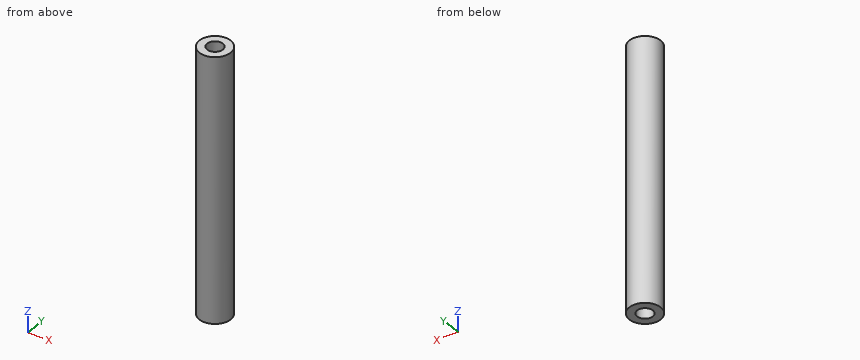
Autodesk Inventor part; units mm, degrees
ref_plane "作業平面1" through (0, 0, 44) normal (0, 0, 1) x (1, 0, 0)
ref_plane "YZ Plane" through (0, 0, 0) normal (1, 0, 0) x (0, 1, 0)
ref_plane "XZ Plane" through (0, 0, 0) normal (0, 1, 0) x (-1, 0, 0)
sketch "スケッチ1" plane through (0, 0, 0) normal (0, 0, 1) x (1, 0, 0)
  circle A0 centre (0, 0) radius 1.5
  circle A1 centre (0, 0) radius 3
  dimension "d0" = 3
  dimension "d1" = 6
extrude "押し出し1" add sketch "スケッチ1" along normal blind 50
ref_plane "作業平面1" through (0, 0, 44) normal (0, 0, 1) x (1, 0, 0)
sketch "スケッチ3" plane through (0, 0, 44) normal (0, 0, 1) x (1, 0, 0)
  circle A0 centre (0, 0) radius 1.5
extrude "押し出し3" add sketch "スケッチ3" against normal blind 38
properties part number "スペーサーm3,50" material "アルミニウム 7075"
Here's how the part is built. I have some questions about the finished solid (model axes, mm). Give positions to 0.01 mm unless a question says otherwise; leave off trailing zeros. Order: outer loops, then holes, each group sorted by start corner. A loop starts at its lowest first (then second) coordinate and runs counter-clockwise, first axis right, second up. Notation, with made-up numbers: (43.25, 70) -> (93.25, 70) arc R4 cw to (93.25, 75) -> close; hole circle Ø6 at (11.25, -18). An arc over 180 degrees is marked (long way). One line per item, written item: value. Start each with the question number.
1. I need wall thicknesses on probe 1 along Y at (x, z) = (0, 46.6); probe 2 along X at (y, z) = (0.25, 10.5); probe 3 along Z at (x, y) = (1.05, 0.1). Which ranges of each line are inside material? Lowest first, please. Write a range as from..to.
2. Imagine slicing it at C-C, the plane z = 41. List the corners of the cut face in (x, y) for me, plus the area to 3 significant figures.
3. Imagine slicing it at A-A, the plane x = 0. List the corners of the cut face in (y, z) for me, plus the area to 3 significant figures.
4. Will these pins go through, and if not, where does the flat tip stop? pin 1 Ø0.9 at (x, y) = (0, 0.5) entering from +Z; pin 2 Ø1 at (y, z) = (-2, 20) entering from +X; pin 3 Ø2 at (y, z) = (-1.5, 34.5) entering from -X.
5. Imagine slicing it at D-D, the plane x = -2.45. List the corners of the cut face in (y, z) for me, plus the area to 3 significant figures.
Values follow:
1. probe 1: y = -3..-1.5, 1.5..3
1. probe 2: x = -2.99..2.99
1. probe 3: z = 6..44
2. outline: circle Ø6 at (0, 0)
2. area: 28.3 mm2
3. outline: (-3, 0) -> (-1.5, 0) -> (-1.5, 6) -> (1.5, 6) -> (1.5, 0) -> (3, 0) -> (3, 50) -> (1.5, 50) -> (1.5, 44) -> (-1.5, 44) -> (-1.5, 50) -> (-3, 50) -> close
3. area: 264 mm2
4. pin 1: stops at z = 44
4. pin 2: stops at x = 2.6
4. pin 3: stops at x = -2.96
5. outline: (-1.73, 0) -> (1.73, 0) -> (1.73, 50) -> (-1.73, 50) -> close
5. area: 173 mm2
